Source: CAD feature listing. Evaluate the final solid. Frame: model axes, mm. Face numbers are marked on the shaded views. A direction names the side the tool comes from. Coordinates: 2 decimals unless noted, no trailing zeros. Write each loop counter-clockwise with the first axis right and the second up, starting at its lowest first coordinate (ties: lowest second). Pieces come first, ordered by that corner, then holes. Notation, with made-up numbers: (17, 46) -> (46, 46) arc R20 cw to (46, 53) -> close; hole circle Ø9 at (-27, 75). An arc over 180 degrees is marked (long way). Write item = value, one per line.
from build123d import *

# Parameters (mm, degrees)
SKETCH2_W           = 108
SKETCH2_H           = 70
SKETCH2_R           = 2.25
BOSS_EXTRUDE1_DEPTH = 3
SKETCH5_R           = 3.5635
SKETCH5_R_2         = 1.8135
BOSS_EXTRUDE2_DEPTH = 5
SKETCH6_R           = 1.8135
BOSS_EXTRUDE3_DEPTH = 2
SKETCH7_W           = 108
SKETCH7_H           = 70
SKETCH7_W_2         = 102
SKETCH7_H_2         = 64
BOSS_EXTRUDE4_DEPTH = 6.65
SKETCH9_W           = 89.35
SKETCH9_H           = 3
CUT_EXTRUDE1_DEPTH  = 1.5
SKETCH11_W          = 12
SKETCH11_H          = 18
SKETCH11_R          = 3.25
BOSS_EXTRUDE5_DEPTH = 9.65
FILLET1_R           = 2
SKETCH12_R          = 5.5
CUT_EXTRUDE2_DEPTH  = 6.2


with BuildPart() as part:
    # Sketch2 → Boss-Extrude1 (new body)
    with BuildSketch(Plane(origin=(0, 0, 0), x_dir=(1, 0, 0), z_dir=(0, 1, 0))):
        with Locations((-7.231065886, 6.378485879)):
            Rectangle(SKETCH2_W, SKETCH2_H)
        with Locations(Location((20.268934114, 4.878485879, 0), (0, 0, 270))):
            Circle(SKETCH2_R, mode=Mode.SUBTRACT)
        with Locations(Location((10.268934114, 4.878485879, 0), (0, 0, 270))):
            Circle(SKETCH2_R, mode=Mode.SUBTRACT)
        with Locations(Location((0.268934114, 4.878485879, 0), (0, 0, 270))):
            Circle(SKETCH2_R, mode=Mode.SUBTRACT)
        with Locations(Location((10.268934114, 12.878485879, 0), (0, 0, 270))):
            Circle(SKETCH2_R, mode=Mode.SUBTRACT)
        with Locations(Location((0.268934114, 12.878485879, 0), (0, 0, 270))):
            Circle(SKETCH2_R, mode=Mode.SUBTRACT)
        with Locations(Location((10.268934114, 20.878485879, 0), (0, 0, 270))):
            Circle(SKETCH2_R, mode=Mode.SUBTRACT)
        with Locations(Location((0.268934114, 20.878485879, 0), (0, 0, 270))):
            Circle(SKETCH2_R, mode=Mode.SUBTRACT)
        with Locations(Location((20.268934114, 12.878485879, 0), (0, 0, 270))):
            Circle(SKETCH2_R, mode=Mode.SUBTRACT)
        with Locations(Location((20.268934114, 20.878485879, 0), (0, 0, 270))):
            Circle(SKETCH2_R, mode=Mode.SUBTRACT)
        with Locations(Location((-9.731065886, 4.878485879, 0), (0, 0, 270))):
            Circle(SKETCH2_R, mode=Mode.SUBTRACT)
        with Locations(Location((-9.731065886, 12.878485879, 0), (0, 0, 270))):
            Circle(SKETCH2_R, mode=Mode.SUBTRACT)
        with Locations(Location((-9.731065886, 20.878485879, 0), (0, 0, 270))):
            Circle(SKETCH2_R, mode=Mode.SUBTRACT)
        with Locations(Location((-19.731065886, 4.878485879, 0), (0, 0, 270))):
            Circle(SKETCH2_R, mode=Mode.SUBTRACT)
        with Locations(Location((-19.731065886, 12.878485879, 0), (0, 0, 270))):
            Circle(SKETCH2_R, mode=Mode.SUBTRACT)
        with Locations(Location((-19.731065886, 20.878485879, 0), (0, 0, 270))):
            Circle(SKETCH2_R, mode=Mode.SUBTRACT)
    extrude(amount=-BOSS_EXTRUDE1_DEPTH)

    # Sketch5 → Boss-Extrude2 (add)
    # profile 1 of 4: a face of its own
    with BuildSketch(Plane(origin=(0, 0, 0), x_dir=(1, 0, 0), z_dir=(0, 1, 0))):
        with Locations(Location((-37.231065886, 32.378485879, 0), (0, 0, 270))):
            Circle(SKETCH5_R)
        with Locations(Location((-37.231065886, 32.378485879, 0), (0, 0, 270))):
            Circle(SKETCH5_R_2, mode=Mode.SUBTRACT)
    # profile 2 of 4: a face of its own
    with BuildSketch(Plane(origin=(0, 0, 0), x_dir=(1, 0, 0), z_dir=(0, 1, 0))):
        with Locations(Location((37.768934114, 32.378485879, 0), (0, 0, 270))):
            Circle(SKETCH5_R)
        with Locations(Location((37.768934114, 32.378485879, 0), (0, 0, 270))):
            Circle(SKETCH5_R_2, mode=Mode.SUBTRACT)
    # profile 3 of 4: a face of its own
    with BuildSketch(Plane(origin=(0, 0, 0), x_dir=(1, 0, 0), z_dir=(0, 1, 0))):
        with Locations(Location((37.768934114, -6.621514121, 0), (0, 0, 270))):
            Circle(SKETCH5_R)
        with Locations(Location((37.768934114, -6.621514121, 0), (0, 0, 270))):
            Circle(SKETCH5_R_2, mode=Mode.SUBTRACT)
    # profile 4 of 4: a face of its own
    with BuildSketch(Plane(origin=(0, 0, 0), x_dir=(1, 0, 0), z_dir=(0, 1, 0))):
        with Locations(Location((-37.231065886, -6.621514121, 0), (0, 0, 270))):
            Circle(SKETCH5_R)
        with Locations(Location((-37.231065886, -6.621514121, 0), (0, 0, 270))):
            Circle(SKETCH5_R_2, mode=Mode.SUBTRACT)
    extrude(amount=BOSS_EXTRUDE2_DEPTH)

    # Sketch6 → Boss-Extrude3 (add)
    with BuildSketch(Plane(origin=(0, 0, 0), x_dir=(1, 0, 0), z_dir=(0, 1, 0))):
        with Locations(Location((-37.231065886, 32.378485879, 0), (0, 0, 270))):
            Circle(SKETCH6_R)
        with Locations(Location((37.768934114, 32.378485879, 0), (0, 0, 270))):
            Circle(SKETCH6_R)
        with Locations(Location((37.768934114, -6.621514121, 0), (0, 0, 270))):
            Circle(SKETCH6_R)
        with Locations(Location((-37.231065886, -6.621514121, 0), (0, 0, 270))):
            Circle(SKETCH6_R)
    extrude(amount=BOSS_EXTRUDE3_DEPTH)

    # Sketch7 → Boss-Extrude4 (add)
    with BuildSketch(Plane(origin=(0, 0, 0), x_dir=(1, 0, 0), z_dir=(0, 1, 0))):
        with Locations((-7.231065886, 6.378485879)):
            Rectangle(SKETCH7_W, SKETCH7_H)
        with Locations((-7.231065886, 6.378485879)):
            Rectangle(SKETCH7_W_2, SKETCH7_H_2, mode=Mode.SUBTRACT)
    extrude(amount=BOSS_EXTRUDE4_DEPTH)

    # Sketch9 → Cut-Extrude1 (cut)
    with BuildSketch(Plane(origin=(0, 6.65, 0), x_dir=(1, 0, 0), z_dir=(0, 1, 0))):
        with Locations((-7.106065886, -27.121514121)):
            Rectangle(SKETCH9_W, SKETCH9_H)
    extrude(amount=-CUT_EXTRUDE1_DEPTH, mode=Mode.SUBTRACT)

    # Sketch11 → Boss-Extrude5 (add)
    # profile 1 of 2: a face of its own
    with BuildSketch(Plane.XZ.offset(3)):
        with Locations((-67.231065886, -6.378485879)):
            Rectangle(SKETCH11_W, SKETCH11_H)
        with Locations(Location((-65.731065886, -6.378485879, 0), (0, 0, 270))):
            Circle(SKETCH11_R, mode=Mode.SUBTRACT)
    # profile 2 of 2: a face of its own
    with BuildSketch(Plane.XZ.offset(3)):
        with Locations((52.768934114, -6.378485879)):
            Rectangle(SKETCH11_W, SKETCH11_H)
        with Locations(Location((51.268934114, -6.378485879, 0), (0, 0, 90))):
            Circle(SKETCH11_R, mode=Mode.SUBTRACT)
    extrude(amount=-BOSS_EXTRUDE5_DEPTH)

    # Fillet1
    fillet1_edges = [part.edges().sort_by_distance(p)[0] for p in [
        (-73.231065886, 1.825, -15.378485879),
        (-73.231065886, 1.825, 2.621514121),
        (58.768934114, 1.825, 2.621514121),
        (58.768934114, 1.825, -15.378485879),
    ]]
    fillet(fillet1_edges, radius=FILLET1_R)

    # Sketch12 → Cut-Extrude2 (cut)
    with BuildSketch(Plane.XZ.offset(3)):
        with Locations(Location((-65.731065886, -6.378485879, 0), (0, 0, 270))):
            Circle(SKETCH12_R)
        with Locations(Location((51.268934114, -6.378485879, 0), (0, 0, 270))):
            Circle(SKETCH12_R)
    extrude(amount=-CUT_EXTRUDE2_DEPTH, mode=Mode.SUBTRACT)


solid = part.part
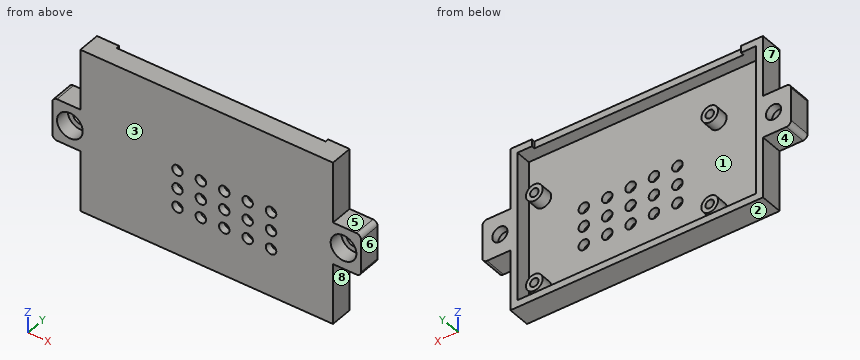
1) Cut plane B-B, the plane x = -50. Output: boundary loops of the cut face in (y, z), and give its area (3 significant figures).
Answer block:
outline = (-3, -41.38) -> (6.65, -41.38) -> (6.65, -38.38) -> (0, -38.38) -> (0, 25.62) -> (5.15, 25.62) -> (5.15, 28.62) -> (-3, 28.62) -> close
area = 245 mm2
2) Material intervals for probe 1 along Z at (x, y) = (0.5, 1); probe 2 along X at (y, z) = (5.5, 5); probe 3 along X at (y, z) = (0.5, -9.5), sorted ascending. Write a range as [from, to].
Answer block:
probe_1 = [-41.38, -38.38], [25.62, 28.62]
probe_2 = [-61.23, -58.23], [43.77, 46.77]
probe_3 = [-73.23, -70.26], [-61.2, -58.23], [43.77, 46.74], [55.8, 58.77]
3) Cut plane D-D, the plane x = -64. Output: boundary loops of the cut face in (y, z), and give its area (3 significant figures).
Answer block:
outline = (-3, -15.38) -> (6.65, -15.38) -> (6.65, -9.13) -> (3.2, -9.13) -> (3.2, -11.6) -> (-3, -11.6) -> close; (-3, -1.16) -> (3.2, -1.16) -> (3.2, -3.63) -> (6.65, -3.63) -> (6.65, 2.62) -> (-3, 2.62) -> close
area = 90.0 mm2
4) Pull-direction query (Z, two-part tool) for the marked faces 1, 2 and 3; classes: +Z half, -Z half, draft (parallel to the pull), parting line (faces both ways), or undercut.
Answer block:
face_1 = undercut
face_2 = -Z half
face_3 = draft
5) Cut plane C-C, the plane y = -1.25. Give the number of separate pieces and of enclosed holes in the cut face, and give its area (3 significant figures).
Answer block:
separate_pieces = 1
enclosed_holes = 17
area = 7,560 mm2
6) Cut plane A-A, the plane z = 15. Output: boundary loops of the cut face in (x, y), and give its area (3 significant figures).
Answer block:
outline = (-61.23, -3) -> (46.77, -3) -> (46.77, 6.65) -> (43.77, 6.65) -> (43.77, 0) -> (-58.23, 0) -> (-58.23, 6.65) -> (-61.23, 6.65) -> close
area = 364 mm2
7) First-contact query: pin 1 Ø5 at (y, z) = (0.5, 21.5) entering from +X; pin 2 Ø1 at (y, z) = (0.5, 12.5) entering from -X; pin 3 Ø1.5 at (x, z) = (3.5, -22) entering from +Y. Flat tips, straight axial feed; report the tip coordinate or a pass-through.
Answer block:
pin_1 = 46.77
pin_2 = -61.23
pin_3 = 0
8) Reachability of the marked faces 4, 5, 6, 7 and 8 from +Z, -Z, +X, -X, +Y, -Y: full face, straight path, thin tool, end or side. Return the list, or none.
Answer block:
face_4 = -Z, -X, +Y, -Y
face_5 = +Z, +X, +Y, -Y
face_6 = +Z, -Z, +X, +Y, -Y
face_7 = +Z, -X, +Y, -Y
face_8 = -Z, +X, +Y, -Y
